Model file for the job. Use its own axes, mm. Face numbers are marked on the shaded views. A direction names the side the tool comes from. Round coordinates to 2 decimals unless told otherwise and drop trailing zeros. Order: outer loops, then holes, each group sorted by start corner. A loop starts at its lowest first (then second) coordinate and runs counter-clockwise, first axis right, second up. Notation, with made-up numbers: (27.25, 75) - (79.25, 75) arc R8 ccw to (79.25, 90) - close; hole circle Ø4 at (-5, 57). An arc over 180 degrees is marked (long way). Answer as CSV lines item,"result". Start each with the question number.
1. 3-axis set-ups, long thin cutter, end or side, ignore diameter. For the marked faces 1 and 2: which of +Z, -Z, +X, -X, +Y, -Y reach the whole face in a straight line?
2. Band-saw the part on A-A on z = 0. List the corners of the cut face in (x, y).
3. Pull direction Z, two halves, no side cores. Call the marked faces 3 and 4: released by +Z, released by -Z, zero draft, split by the parting line, or undercut.
4. Pin check, flat tip, straight feed: pin 1 Ø6 at (x, z) = (-4, -3) entering from +Y. Stop position of the tip, or through.
5. Band-saw the part on D-D on z = 7.75. List the corners of the cut face in (x, y), then the cut area to 3 significant figures.
6. Band-saw the part on C-C on y = 0.7. State how many separate pieces and enclosed holes the cut face has, then the cut area to 3 significant figures.
7. Wall check: line 1 along X through (y, z) = (1.25, 0); line 2 along Z through (x, y) = (-4.75, 0.45); line 3 along Z through (x, y) = (3, 0.8). Give the ranges that are in metal, low to high. Write a range as [from, to].
8. Band-saw the part on B-B on x = -3. List the corners of the cut face in (y, z).
Autodesk Inventor part; units mm, degrees
ref_plane "YZ Plane" through (0, 0, 0) normal (1, 0, 0) x (0, 1, 0)
ref_plane "XZ Plane" through (0, 0, 0) normal (0, 1, 0) x (-1, 0, 0)
ref_plane "XY Plane" through (0, 0, 0) normal (0, 0, 1) x (1, 0, 0)
sketch "スケッチ1" plane through (0, 0, 0) normal (0, 1, 0) x (-1, 0, 0)
  circle A0 centre (0, 0) radius 9.5
  dimension "d0" = 19
extrude "押し出し1" add sketch "スケッチ1" along normal blind 1
sketch "スケッチ2" plane through (0, 1, 0) normal (0, 1, 0) x (1, 0, 0)
  circle A0 centre (0, 0) radius 8
  dimension "d4" = 16
extrude "押し出し2" add sketch "スケッチ2" along normal blind 1
sketch "スケッチ4" plane through (0, 2, 0) normal (0, 1, 0) x (1, 0, 0)
  circle A0 centre (0, 0) radius 3.5
  dimension "d20" = 7
extrude "押し出し4" cut sketch "スケッチ4" against normal blind 10
sketch "スケッチ5" plane through (0, 2, 0) normal (0, 1, 0) x (1, 0, 0)
  arc A0 (1.5668, 6.4373) -> (0, 6.5319) centre (0.7805, 6.4373) ccw
  arc A1 (0, 4.2235) -> (1.5668, 6.4373) centre (-0.7805, 6.4373) ccw
  line L0 (0, 6.5319) -> (0, 4.2235)
  line L1 (0.7805, 6.4373) -> (0, 6.4373) construction
  line L2 (-0.7805, 6.4373) -> (0, 6.4373) construction
  line L3 (1.5668, 4.5823) -> (1.5668, 2.8488) construction
  line L4 (1.5668, 5.2864) -> (1.5668, 3.0604) construction
  line L5 (-0.8113, 7.2235) -> (2.563, 7.2235) construction
  line L6 (0.8759, 7.2235) -> (0.963, 7.9418) construction
  line L7 (0, 4.2235) -> (0, 3.5) construction
  circle A2 centre (0, 0) radius 3.5 construction
  circle A3 centre (0, 0) radius 8 construction
  line L8 (-0.0717, 5.941) -> (0.1752, 7.9769) construction
  arc A4 (0, 6.5319) -> (-1.5668, 6.4373) centre (-0.7805, 6.4373) ccw
  arc A5 (-1.5668, 6.4373) -> (0, 4.2235) centre (0.7805, 6.4373) ccw
  circle A6 centre (3, 5.1962) radius 0.75
  circle A7 centre (0, 0) radius 6 construction
  dimension "d33" = 12
  dimension "d24" = 3
  dimension "d31" = 1.5
  dimension "d32" = 30
extrude "押し出し5" cut sketch "スケッチ5" against normal blind 10
fillet "フィレット1" radius 0.5 2 edges at (0, 1, -6.5319) (0, 1, -4.2235)
pattern_circular "円形状パターン1" count 6 over 360 about axis through (0, -10, 0) along (0, 1, 0) of "押し出し5", "フィレット1"
properties part number "wheelcap" material "ABS プラスチック"
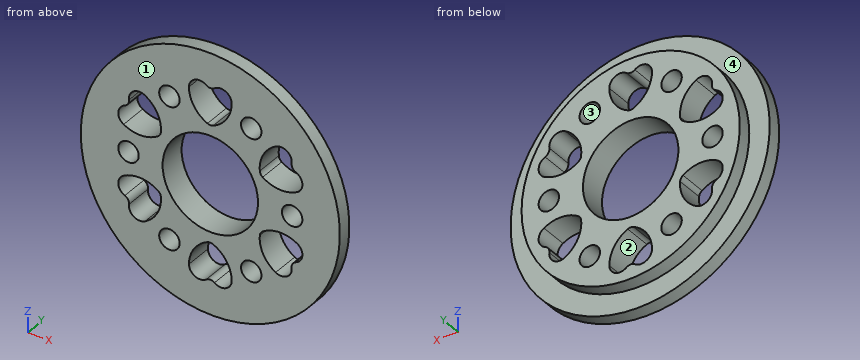
Reply:
1,face 1,"+Z, -Z, +X, -X, -Y"
1,face 2,"+Y, -Y"
2,outline,"(-9.5, 0) - (-6.75, 0) - (-6.75, 2) - (-8, 2) - (-8, 1) - (-9.5, 1) - close; (-5.25, 0) - (-3.5, 0) - (-3.5, 2) - (-5.25, 2) - close; (3.5, 0) - (5.25, 0) - (5.25, 2) - (3.5, 2) - close; (6.75, 0) - (9.5, 0) - (9.5, 1) - (8, 1) - (8, 2) - (6.75, 2) - close"
3,face 3,"undercut"
3,face 4,"zero draft"
4,pin 1,"stops at y = 2"
5,outline,"(-5.49, 0) - (5.49, 0) - (5.49, 1) - (1.98, 1) - (1.98, 2) - (-1.98, 2) - (-1.98, 1) - (-5.49, 1) - close"
5,area,"15.0 mm2"
6,separate pieces,"1"
6,enclosed holes,"13"
6,area,"192 mm2"
7,line 1,"x = [-8, -6.75], [-5.25, -3.5], [3.5, 5.25], [6.75, 8]"
7,line 2,"z = [-8.23, -4.55], [-1.59, 1.59], [4.55, 8.23]"
7,line 3,"z = [-9.01, -5.95], [-4.45, -1.8], [1.8, 4.45], [5.95, 9.01]"
8,outline,"(0, -9.01) - (1, -9.01) - (1, -7.42) - (2, -7.42) - (2, -5.95) - (0, -5.95) - close; (0, -4.45) - (2, -4.45) - (2, -1.8) - (0, -1.8) - close; (0, 1.8) - (2, 1.8) - (2, 4.45) - (0, 4.45) - close; (0, 5.95) - (2, 5.95) - (2, 7.42) - (1, 7.42) - (1, 9.01) - (0, 9.01) - close"
